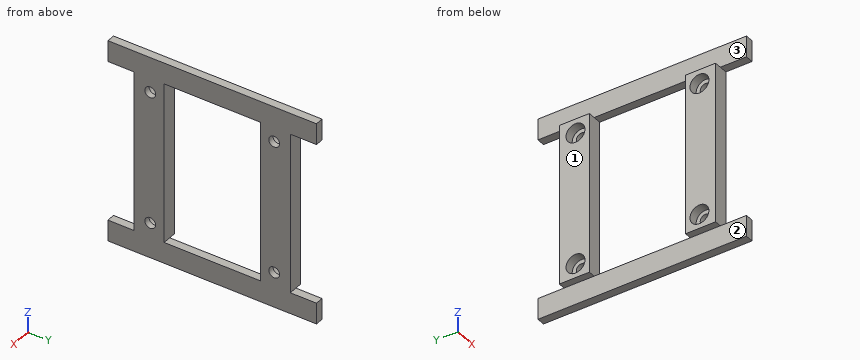
from build123d import *

# Parameters (mm, degrees)
SKETCH1_W             = 7
SKETCH1_H             = 69.4
BOSS_EXTRUDE1_DEPTH   = 2.7
BOSS_EXTRUDE1_2_DEPTH = 2.7
SKETCH1_7_W           = 53.4
SKETCH1_7_H           = 10
SKETCH1_7_R           = 1.8
BOSS_EXTRUDE2_DEPTH   = 5
SKETCH2_R             = 3.15
CUT_EXTRUDE1_DEPTH    = 3


with BuildPart() as part:
    # Sketch1 → Boss-Extrude1 (new body)
    with BuildSketch(Plane(origin=(0, 0, 0), x_dir=(0, 0, -1), z_dir=(1, 0, 0))):
        with Locations((-30.2, 0)):
            Rectangle(SKETCH1_W, SKETCH1_H)
    extrude(amount=-BOSS_EXTRUDE1_DEPTH)



with BuildPart() as body_2:
    # Sketch1 → Boss-Extrude1 2 (new body)
    with BuildSketch(Plane(origin=(0, 0, 0), x_dir=(0, 0, -1), z_dir=(1, 0, 0))):
        with Locations((30.2, 0)):
            Rectangle(SKETCH1_W, SKETCH1_H)
    extrude(amount=-BOSS_EXTRUDE1_2_DEPTH)


with BuildPart() as part_1:
    add(part.part)

    add(body_2.part)  # Boss-Extrude2 merges body 2
    # Sketch1_7 → Boss-Extrude2 (add)
    # profile 1 of 2: a face of its own
    with BuildSketch(Plane(origin=(0, 0, 0), x_dir=(0, 0, -1), z_dir=(1, 0, 0))):
        with Locations((0, 21)):
            Rectangle(SKETCH1_7_W, SKETCH1_7_H)
        with Locations((-22, 20.625876568)):
            Circle(SKETCH1_7_R, mode=Mode.SUBTRACT)
        with Locations(Location((22, 20.625876568, 0), (0, 0, 180))):
            Circle(SKETCH1_7_R, mode=Mode.SUBTRACT)
    # profile 2 of 2: a face of its own
    with BuildSketch(Plane(origin=(0, 0, 0), x_dir=(0, 0, -1), z_dir=(1, 0, 0))):
        with Locations((0, -21)):
            Rectangle(SKETCH1_7_W, SKETCH1_7_H)
        with Locations((22, -20.625876568)):
            Circle(SKETCH1_7_R, mode=Mode.SUBTRACT)
        with Locations(Location((-22, -20.625876568, 0), (0, 0, 180))):
            Circle(SKETCH1_7_R, mode=Mode.SUBTRACT)
    extrude(amount=-BOSS_EXTRUDE2_DEPTH)

    # Sketch2 → Cut-Extrude1 (cut)
    with BuildSketch(Plane.ZY.offset(5)):
        with Locations((-22, 20.625876568)):
            Circle(SKETCH2_R)
        with Locations((22, 20.625876568)):
            Circle(SKETCH2_R)
        with Locations((-22, -20.625876568)):
            Circle(SKETCH2_R)
        with Locations((22, -20.625876568)):
            Circle(SKETCH2_R)
    extrude(amount=-CUT_EXTRUDE1_DEPTH, mode=Mode.SUBTRACT)


solid = part_1.part
Source: CAD feature listing. Evaluate the final solid. Frame: model axes, mm. Face numbers are marked on the shaded views. A direction names the side the tool comes from. Coordinates: 2 decimals unless noted, no trailing zeros. Order: outer loops, then holes, each group sorted by start corner. A loop starts at its lowest first (then second) coordinate and runs counter-clockwise, first axis right, second up. Notation, with made-up numbers: M 73,15 L 88,15 A19 ccw 88,48 Z; hole C -10.5,-12.75 d11. An arc over 180 degrees is marked long. Write each question's results on one line, items separated by ' | '. Start each with the question number.
1. Section A-A, the plane z = 22. Return the cut outline in (x, y).
2. Section D-D, the plane y = 9. Return the cut outline in (x, z), then the cut area to 3 significant figures.
3. Section B-B, the plane x = -3.9. Return the cut outline in (y, z).
4. Section C-C, the plane z = -0.5. Return the cut outline in (x, y).
5. Pin query (flat end, axial travel): pin 1 (0.7 mm diameter, centred on x = -3.5, y = -22, fed in from -Z); pin 2 (0.7 mm diameter, centred on x = -3.5, y = -20, fed in from +Z); pin 3 (1 mm diameter, centred on x = -3.5, z = 11, fed in from -Y); pin 4 (1.9 mm diameter, centred on y = 20.5, z = -22.5, fed in from -X). Return the tip coordinate at first contact, or that it passes through.
6. Reachability of the marked faces 1, 2 and 3 from +Z, -Z, +X, -X, +Y, -Y: full face, straight path, thin tool, end or side. Return the list, or none.
7. Material intervals for L1, parallel to Y at x = -4.4, z = -22; L2, parallel to Y at x = -1.5, z = 22; L3, parallel to Z at x = -2.6, y = 0, sorted ascending.
Solution:
1) outline: M -5,-26 L 0,-26 L 0,-22.43 L -2,-22.43 L -2,-23.78 L -5,-23.78 Z; M -5,-17.48 L -2,-17.48 L -2,-18.83 L 0,-18.83 L 0,-16 L -5,-16 Z; M -5,16 L 0,16 L 0,18.83 L -2,18.83 L -2,17.48 L -5,17.48 Z; M -5,23.78 L -2,23.78 L -2,22.43 L 0,22.43 L 0,26 L -5,26 Z
2) outline: M -2.7,-33.7 L 0,-33.7 L 0,-26.7 L -2.7,-26.7 Z; M -2.7,26.7 L 0,26.7 L 0,33.7 L -2.7,33.7 Z | area: 37.8 mm²
3) outline: M -26,-26.7 L -16,-26.7 L -16,26.7 L -26,26.7 Z; M 16,-26.7 L 26,-26.7 L 26,26.7 L 16,26.7 Z; hole C -20.63,-22 d6.3; hole C -20.63,22 d6.3; hole C 20.63,-22 d6.3; hole C 20.63,22 d6.3
4) outline: M -5,-26 L 0,-26 L 0,-16 L -5,-16 Z; M -5,16 L 0,16 L 0,26 L -5,26 Z
5) pin 1: z = -26.7 | pin 2: z = 26.7 | pin 3: y = -26 | pin 4: through
6) face 1: +Z, -Z, -X, +Y, -Y | face 2: -Z, -X, +Y, -Y | face 3: +Z, -X, +Y, -Y
7) L1: -26 to -23.78, -17.48 to -16, 16 to 17.48, 23.78 to 26 | L2: -26 to -22.43, -18.83 to -16, 16 to 18.83, 22.43 to 26 | L3: -33.7 to -26.7, 26.7 to 33.7
